from build123d import *

# Parameters (mm, degrees)
CYLINDER_R        = 29.5
CYLINDER_DEPTH    = 150
BOX_W             = 35
BOX_H             = 50
BOX_DEPTH         = 132
CYLINDER001_R     = 10
CYLINDER001_DEPTH = 3
PRISM_DEPTH       = 7


with BuildPart() as part:
    # Cylinder → Cylinder (join)
    with BuildSketch(Plane.XY):
        Circle(CYLINDER_R)
    extrude(amount=CYLINDER_DEPTH)

    # Box → Box (cut)
    with BuildSketch(Plane(origin=(-17.5, -17.5, 10), x_dir=(1, 0, 0), z_dir=(0, 0, 1))):
        with Locations((17.5, 25)):
            Rectangle(BOX_W, BOX_H)
    extrude(amount=BOX_DEPTH, mode=Mode.SUBTRACT)

    # Cylinder001 → Cylinder001 (join)
    with BuildSketch(Plane.XY.offset(150)):
        Circle(CYLINDER001_R)
    extrude(amount=CYLINDER001_DEPTH)

    # Prism → Prism (join)
    with BuildSketch(Plane.XY.offset(153)):
        Polygon((10, 0), (5, 8.660254), (-5, 8.660254), (-10, 0), (-5, -8.660254), (5, -8.660254), align=None)
    extrude(amount=PRISM_DEPTH)


solid = part.part
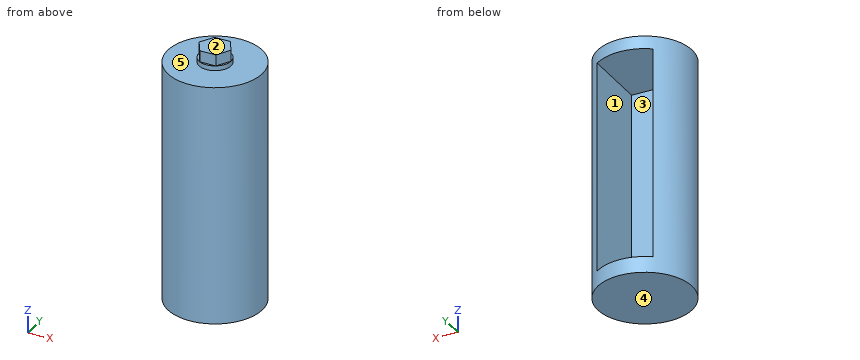
Can you work these out from the model? Positions are in its coordinate system, mm. Face numbers are marked on the shaded views. A direction names the side the tool comes from. Give positions to 0.01 mm unless a question says otherwise; leave off trailing zeros. Loops run counter-clockwise (first coordinate to the right, second up) from the corner with the lowest first, then second, coordinate; pieces in that order, holes last. Notation, with made-up numbers: (52, 61.5) - (63, 61.5) arc R21 ccw to (63, 90.5) - close; hole circle Ø1 at (-38, 4). An arc over 180 degrees is marked (long way). Return JSON: item names as keys, results as strings.
1. I want a section at D-D on y = -25. Please give me the cut outline in (x, z), and give its area (3 significant figures).
Output values:
{"outline": "(-15.66, 0) - (15.66, 0) - (15.66, 150) - (-15.66, 150) - close", "area": "4,700 mm²"}
2. I want a section at A-A on x = 0. Please give me the cut outline in (y, z), and give its area (3 significant figures).
Output values:
{"outline": "(-29.5, 0) - (29.5, 0) - (29.5, 10) - (-17.5, 10) - (-17.5, 142) - (29.5, 142) - (29.5, 150) - (10, 150) - (10, 153) - (8.66, 153) - (8.66, 160) - (-8.66, 160) - (-8.66, 153) - (-10, 153) - (-10, 150) - (-29.5, 150) - close", "area": "2,830 mm²"}
3. I want a section at C-C on x = -15. Please give me the cut outline in (y, z), and give its area (3 significant figures).
Output values:
{"outline": "(-25.4, 0) - (25.4, 0) - (25.4, 10) - (-17.5, 10) - (-17.5, 142) - (25.4, 142) - (25.4, 150) - (-25.4, 150) - close", "area": "1,960 mm²"}
4. I want a section at B-B on z = 62. Please give me the cut outline in (x, y), and give its area (3 significant figures).
Output values:
{"outline": "(-17.5, -17.5) - (-17.5, 23.75) arc R29.5 ccw (long way) to (17.5, 23.75) - (17.5, -17.5) - close", "area": "1,150 mm²"}
5. If I drill on line 1 (Z direction, x = 4, y = -15); line 2 (Z direction, x = -19.5, y = 1); line 3 (X direction, y = 19.5, z = 109), over which ranges is the centre line in solid material (lowest first)?
Output values:
{"line 1": "z = 0 to 10, 142 to 150", "line 2": "z = 0 to 150", "line 3": "x = -22.14 to -17.5, 17.5 to 22.14"}
6. We'd pull the mould along Z, two halves only. Please class the marked faces 3, 4 and 5: +Z half, -Z half, draft (parallel to the pull), parting line (faces both ways), or undercut.
Output values:
{"face 3": "undercut", "face 4": "-Z half", "face 5": "+Z half"}
7. For the marked faces 1 and 2, which set-ups out of +Z, -Z, +X, -X, +Y, -Y let a thin tool reach every point of the face, with its end or its side?
Output values:
{"face 1": "+Y", "face 2": "+Z, +X, -X, +Y, -Y"}
8. I'm going to push flat-ended pins straight in: pin 1 Ø1.5 at (x, y) = (-1, 9) entering from +Z; pin 2 Ø2 at (x, z) = (10, 22.5) entering from -Y; pin 3 Ø1.5 at (x, z) = (15, 134.5) entering from +Y; pin 4 Ø6 at (x, y) = (14, 10.5) entering from +Z. Where does each tip first touch, or does it pass through?
Output values:
{"pin 1": "stops at z = 160", "pin 2": "stops at y = -28.09", "pin 3": "stops at y = -17.5", "pin 4": "stops at z = 150"}
